```python
from build123d import *

# Parameters (mm, degrees)
STRUCTURESKETCH001_W      = 192
STRUCTURESKETCH001_H      = 56
MAINSTRUCTURE001_DEPTH    = 81
OBJ1           = 3
CENTERPOCKET001_DEPTH     = 81
OBJ2       = 60
OBJ3       = 50
OBJ4 = 78


with BuildPart() as part:
    # StructureSketch001 → MainStructure001 (new body)
    with BuildSketch(Plane.XY):
        Rectangle(STRUCTURESKETCH001_W, STRUCTURESKETCH001_H)
    extrude(amount=MAINSTRUCTURE001_DEPTH)

    with BuildSketch(Plane(origin=(63, 0, 0), x_dir=(1, 0, 0), z_dir=(0, 0, 1))):
        with Locations((-26, 21)):
            Circle(OBJ1)
        with Locations((26, 21)):
            Circle(OBJ1)
        with Locations((26, -21)):
            Circle(OBJ1)
        with Locations((-26, -21)):
            Circle(OBJ1)
        Polygon((-15, 25), (15, 25), (30, 10), (30, -10), (15, -25), (-15, -25), (-30, -10), (-30, 10), align=None)
    extrude(amount=CENTERPOCKET001_DEPTH, mode=Mode.SUBTRACT)

    with BuildSketch(Plane(origin=(63, 0, 0), x_dir=(1, 0, 0), z_dir=(0, 0, 1))):
        Rectangle(OBJ2, OBJ3)
    extrude(amount=OBJ4, mode=Mode.SUBTRACT)


solid = part.part
```
Geometry: final body of the model. Coordinates: model frame, mm. A direction names the side the tool comes from. Give positions to 0.01 mm unless a question says otherwise; leave off trailing zeros. Loops run counter-clockwise (first coordinate to the right, second up) from the corner with the lowest first, then second, coordinate; pieces in that order, holes last. Notation, with made-up numbers: (82.5, 19) - (141.5, 19) arc R17 ccw to (141.5, 45) - close; hole circle Ø1 at (44.25, 53). An arc over 180 degrees is marked (long way). Answer as CSV lines item,"result". Start each with the question number.
(1) Ray query, line 1 along X through (y, z) = (-8.5, 44); line 2 along Y through (x, z) = (45.5, 17.5); line 3 along X through (y, z) = (21, 79). Return the intervals inside material, ascending. Write a range as [from, to].
(2) Section query A-A (x = 89). Output: boundary loops of the cut face in (y, z), and give its area (3 significant figures).
(3) Reachability of faces 4 (the face through (-23, 0, 81)), 5 (the face through (93, 0, 40)), 6 (the face through (40, 17, 79)) from +Z, -Z, +X, -X, +Y, -Y: full face, straight path, thin tool, end or side. Return the list, or none.
(4) Section query C-C (x = 44). Output: boundary loops of the cut face in (y, z), and give its area (3 significant figures).
(5) Pin query (flat end, axial travel): P1, Ø12, axis at x = 42, y = 14.5, coming from the -Z side; P2, Ø6, axis at x = 6.5, y = 6, coming from the -Z side; P3, Ø3.5, axis at x = 37, y = 21, coming from the +Z side. Return the tip coordinate at first contact, or that it passes through.
(6) Section query B-B (y = -21). Output: boundary loops of the cut face in (x, z), and give its area (3 significant figures).
(7) Section query D-D (z = 63.5). Output: boundary loops of the cut face in (x, y), and give its area (3 significant figures).
(8) Mould query, pull axis X, two halves, no side actions, for faces 1 (the face through (41, -18, 79)), 2 (the face through (-1, -28, 40)), 3 (the face through (-96, 0, 40)). Classes: +X half, -X half, draft (parallel to the pull), parting line (faces both ways), or undercut.
Worked answers:
1,line 1,"x = [-96, 33], [93, 96]"
1,line 2,"y = [-28, -25], [25, 28]"
1,line 3,"x = [-96, 34], [40, 44], [82, 86], [92, 96]"
2,outline,"(-28, 0) - (-25, 0) - (-25, 78) - (-24, 78) - (-24, 81) - (-28, 81) - close; (-18, 78) - (-14, 78) - (-14, 81) - (-18, 81) - close; (14, 78) - (18, 78) - (18, 81) - (14, 81) - close; (24, 78) - (25, 78) - (25, 0) - (28, 0) - (28, 81) - (24, 81) - close"
2,area,"516 mm^2"
3,face 4,"+Z, +X, -X, +Y, -Y"
3,face 5,"-Z"
3,face 6,"+Z, -Z"
4,outline,"(-28, 0) - (-25, 0) - (-25, 78) - (-21, 78) - (-21, 81) - (-28, 81) - close; (21, 78) - (25, 78) - (25, 0) - (28, 0) - (28, 81) - (21, 81) - close"
4,area,"510 mm^2"
5,P1,"stops at z = 78"
5,P2,"stops at z = 0"
5,P3,"passes through"
6,outline,"(-96, 0) - (33, 0) - (33, 78) - (34, 78) - (34, 81) - (-96, 81) - close; (40, 78) - (44, 78) - (44, 81) - (40, 81) - close; (82, 78) - (86, 78) - (86, 81) - (82, 81) - close; (92, 78) - (93, 78) - (93, 0) - (96, 0) - (96, 81) - (92, 81) - close"
6,area,"10,700 mm^2"
7,outline,"(-96, -28) - (96, -28) - (96, 28) - (-96, 28) - close; hole (33, -25) - (93, -25) - (93, 25) - (33, 25) - close"
7,area,"7,750 mm^2"
8,face 1,"undercut"
8,face 2,"draft"
8,face 3,"-X half"
